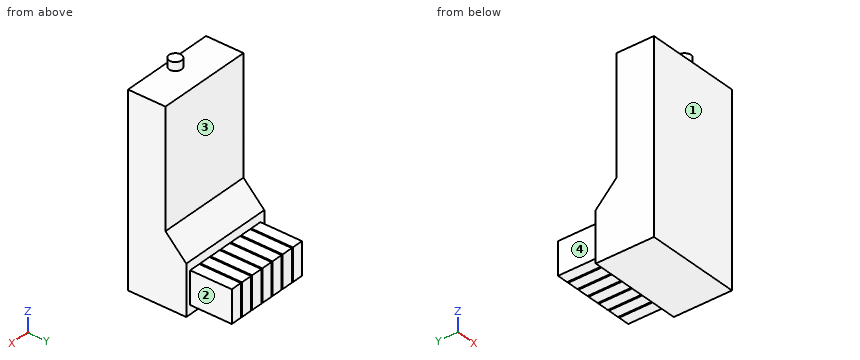
```python
from build123d import *

# Parameters (mm, degrees)
BOSS_EXTRUDE1_DEPTH = 23
SKETCH2_R           = 1.5
BOSS_EXTRUDE2_DEPTH = 2
SKETCH3_W           = 2.7
SKETCH3_H           = 7.8
BOSS_EXTRUDE3_DEPTH = 10


with BuildPart() as part:
    # Sketch1 → Boss-Extrude1 (new body)
    with BuildSketch(Plane(origin=(0, 0, 0), x_dir=(0, 0, -1), z_dir=(1, 0, 0))):
        Polygon((0, 0), (0, 9), (28, 9), (33.16, 14), (45.16, 14), (45.16, 0), align=None)
    extrude(amount=BOSS_EXTRUDE1_DEPTH)

    # Sketch2 → Boss-Extrude2 (add)
    with BuildSketch(Plane.XY):
        with Locations(Location((11.5, 2, 0), (0, 0, 180))):
            Circle(SKETCH2_R)
    extrude(amount=BOSS_EXTRUDE2_DEPTH)

    # Sketch3 → Boss-Extrude3 (add)
    with BuildSketch(Plane(origin=(0, 14, 0), x_dir=(1, 0, 0), z_dir=(0, 1, 0))):
        with Locations((14.5, 39.16)):
            Rectangle(SKETCH3_W, SKETCH3_H)
        with Locations((11.5, 39.16)):
            Rectangle(SKETCH3_W, SKETCH3_H)
        with Locations((17.5, 39.16)):
            Rectangle(SKETCH3_W, SKETCH3_H)
        with Locations((20.5, 39.16)):
            Rectangle(SKETCH3_W, SKETCH3_H)
        with Locations((8.5, 39.16)):
            Rectangle(SKETCH3_W, SKETCH3_H)
        with Locations((5.5, 39.16)):
            Rectangle(SKETCH3_W, SKETCH3_H)
        with Locations((2.5, 39.16)):
            Rectangle(SKETCH3_W, SKETCH3_H)
    extrude(amount=BOSS_EXTRUDE3_DEPTH)


solid = part.part
```
CAD build for the part. Positions are in the model's coordinates, mm. Face numbers are marked on the shaded views. A direction names the side the tool comes from. Round coordinates to 2 decimals unless told otherwise and drop trailing zeros. Loops run counter-clockwise (first coordinate to the right, second up) from the corner with the lowest first, then second, coordinate; pieces in that order, holes last. Notation, with made-up numbers: M 28.25,57.5 L 34.25,57.5 A22 ccw 34.25,79.5 Z; hole C 14.25,-22.75 d9. An arc over 180 degrees is marked long. Return JSON: item names as keys, results as strings. Group by question number.
(1) Tool access for the marked faces 1, 2, 3 and 4: list every direction of +Z, -Z, +X, -X, +Y, -Y with a clear straight run to the whole face (end or side of a thin tool).
(2) Saw through at B-B, the plane x = 11.5. List the corners of the cut face in (y, z).
(3) Saw through at D-D, the plane z = -5.5. List the corners of the cut face in (x, y).
(4) Saw through at C-C, the plane y = 2. List the corners of the cut face in (x, z).
(5) Wall check: probe 1 along Y at (x, z) = (12, -10); probe 2 along Z at (x, y) = (3.5, 4.5); probe 3 along Z at (x, y) = (19.75, 18.5). Give the ranges that are in metal, low to high. Write a range as [from, to].
(6) Saw through at A-A, the plane y = 22.25. List the corners of the cut face in (x, z).
(7) Drop flat-ended pins along their axis: P1, Ø10, axis at x = 15.5, z = -8, coming from the +Y side; P2, Ø0.8, axis at x = 9, y = 21.5, coming from the -Z side; P3, Ø8.5, axis at y = 19.5, z = -39.5, coming from the +X side; P4, Ø5, axis at x = 11, z = -33, coming from the -Y side. Give the stop position or say it passes through.
Answer list:
{
 "1": {"face 1": "+Z, -Z, +X, -X, -Y", "face 2": "+Z, -Z, +X, +Y", "face 3": "+Z, +X, -X, +Y", "face 4": "+Z, -Z, -X, +Y"},
 "2": {"outline": "M 0,-45.16 L 14,-45.16 L 14,-43.06 L 24,-43.06 L 24,-35.26 L 14,-35.26 L 14,-33.16 L 9,-28 L 9,0 L 3.5,0 L 3.5,2 L 0.5,2 L 0.5,0 L 0,0 Z"},
 "3": {"outline": "M 0,0 L 23,0 L 23,9 L 0,9 Z"},
 "4": {"outline": "M 0,-45.16 L 23,-45.16 L 23,0 L 13,0 L 13,2 L 10,2 L 10,0 L 0,0 Z"},
 "5": {"probe 1": "[0, 9]", "probe 2": "[-45.16, 0]", "probe 3": "[-43.06, -35.26]"},
 "6": {"outline": "M 1.15,-43.06 L 3.85,-43.06 L 3.85,-35.26 L 1.15,-35.26 Z; M 4.15,-43.06 L 6.85,-43.06 L 6.85,-35.26 L 4.15,-35.26 Z; M 7.15,-43.06 L 9.85,-43.06 L 9.85,-35.26 L 7.15,-35.26 Z; M 10.15,-43.06 L 12.85,-43.06 L 12.85,-35.26 L 10.15,-35.26 Z; M 13.15,-43.06 L 15.85,-43.06 L 15.85,-35.26 L 13.15,-35.26 Z; M 16.15,-43.06 L 18.85,-43.06 L 18.85,-35.26 L 16.15,-35.26 Z; M 19.15,-43.06 L 21.85,-43.06 L 21.85,-35.26 L 19.15,-35.26 Z"},
 "7": {"P1": "y = 9", "P2": "z = -43.06", "P3": "x = 21.85", "P4": "y = 0"}
}
